CAD build for the part. Positions are in the model's coordinates, mm. A direction names the side the tool comes from. Coordinates: 2 decimals unless noted, no trailing zeros. Write each loop counter-clockwise with the first axis right and the second up, starting at its lowest first coordinate (ties: lowest second). Pieces come first, ordered by that corner, then holes.
```python
from build123d import *

# Parameters (mm, degrees)
BOSS_EXTRUDE1_DEPTH = 10
CUT_EXTRUDE1_DEPTH  = 2
LPATTERN1_COUNT     = 3
LPATTERN1_PITCH     = 2


with BuildPart() as part:
    # Sketch2 → Boss-Extrude1 (new body)
    with BuildSketch(Plane.XY):
        with BuildLine():
            Line((12.25, 1), (12.25, 0.55))
            ThreePointArc((12.25, 0.55), (9.194506694, 0.481441826), (6.145163436, 0.275905297))
            ThreePointArc((6.145163436, 0.275905297), (5.566162178, 0.226280663), (4.986761169, 0.181564549))
            ThreePointArc((4.986761169, 0.181564549), (4.817953434, 0), (4.986761169, -0.181564549))
            ThreePointArc((4.986761169, -0.181564549), (5.566162178, -0.226280663), (6.145163436, -0.275905297))
            ThreePointArc((6.145163436, -0.275905297), (9.194506694, -0.481441826), (12.25, -0.55))
            Line((12.25, -0.55), (12.25, -1))
            ThreePointArc((12.25, -1), (9.174322945, -0.93098895), (6.104836564, -0.724094703))
            ThreePointArc((6.104836564, -0.724094703), (3.055493306, -0.518558174), (0, -0.45))
            ThreePointArc((0, -0.45), (-3.055493306, -0.518558174), (-6.104836564, -0.724094703))
            ThreePointArc((-6.104836564, -0.724094703), (-9.174322945, -0.93098895), (-12.25, -1))
            Line((-12.25, -1), (-12.25, -0.55))
            ThreePointArc((-12.25, -0.55), (-9.194506694, -0.481441826), (-6.145163436, -0.275905297))
            ThreePointArc((-6.145163436, -0.275905297), (-5.566162178, -0.226280663), (-4.986761169, -0.181564549))
            ThreePointArc((-4.986761169, -0.181564549), (-4.817953434, 0), (-4.986761169, 0.181564549))
            ThreePointArc((-4.986761169, 0.181564549), (-5.566162178, 0.226280663), (-6.145163436, 0.275905297))
            ThreePointArc((-6.145163436, 0.275905297), (-9.194506694, 0.481441826), (-12.25, 0.55))
            Line((-12.25, 0.55), (-12.25, 1))
            ThreePointArc((-12.25, 1), (-9.174322945, 0.93098895), (-6.104836564, 0.724094703))
            ThreePointArc((-6.104836564, 0.724094703), (-3.055493306, 0.518558174), (0, 0.45))
            ThreePointArc((0, 0.45), (3.055493306, 0.518558174), (6.104836564, 0.724094703))
            ThreePointArc((6.104836564, 0.724094703), (9.174322945, 0.93098895), (12.25, 1))
        make_face()
    extrude(amount=BOSS_EXTRUDE1_DEPTH)

    # Sketch3 → Cut-Extrude1 (cut, symmetric)
    with BuildSketch(Plane(origin=(0, 0, 0), x_dir=(1, 0, 0), z_dir=(0, 1, 0))):
        Polygon((-2, -3.5), (-1.598076211, -5), (-2, -6.5), (-2.401923789, -5), align=None)
    cut_extrude1 = extrude(amount=CUT_EXTRUDE1_DEPTH, both=True, mode=Mode.SUBTRACT)

    # LPattern1: Cut-Extrude1 ×3
    with Locations(*[(i * LPATTERN1_PITCH, 0, 0) for i in range(1, LPATTERN1_COUNT)]):
        add(cut_extrude1, mode=Mode.SUBTRACT)


solid = part.part
```
Item 1: Flat gauge pins, fed straight in: pin 1 Ø6 at (x, z) = (1, 3.5) entering from -Y; pin 2 Ø1.5 at (x, z) = (1.5, 2) entering from +Y; pin 3 Ø3 at (x, z) = (-7, 1.5) entering from +Y. Where does each tip first touch, or does it go through?
Item 2: Saw through at C-C, the plane z = 7.25. Write the cut outline in (x, y).
Item 3: Wall check: line 1 along Y through (x, z) = (-6, 6); line 2 along Y through (x, z) = (-1.75, 2.5); line 3 along Y through (x, z) = (10, 5). Give the ranges that are in metal, low to high.
Item 4: Saw through at D-D, the plane x = -10. Write the cut outline in (y, z).
Item 5: Saw through at A-A, the plane z = 5.75. State how many separate pieces and enclosed holes the cut face has, and give its area (3 significant figures).
Item 6: Two-plate mould, pull along Z, no slides. Class faces 1 (the flat face through (-0.204, 0.006, 4.26)), 2 (the cylindrical face through (-9.237, -0.483, 4.93)), 3 (the flat face through (0, 0, 0)), 4 (the flat face through (-0.2, 0.01, 5.76)): +Z half, -Z half, draft (parallel to the pull), parting line (faces both ways), or undercut.
Item 7: Saw through at B-B, the plane x = 8.5. Write the cut outline in (y, z), and give its area (3 significant figures).
Item 8: Which spindle directions (+Z, -Z, +X, -X, +Y, -Y) get a long thin tool onto all of the face, cutting with end or side? Do faces 5 (the cylindrical face through (9.217, -0.933, 4.93)), 6 (the cylindrical face through (-9.217, 0.933, 4.93)), 7 (the cylindrical face through (5.574, 0.227, 4.93)). Say none if no direction does.
Working result:
1. pin 1: stops at y = -0.57
1. pin 2: stops at y = 0.49
1. pin 3: stops at y = 0.9
2. outline: (-12.25, -1) arc R68.57 ccw to (-6.1, -0.72) arc R68.12 cw to (6.1, -0.72) arc R68.57 ccw to (12.25, -1) - (12.25, -0.55) arc R68.12 cw to (6.15, -0.28) arc R68.57 ccw to (4.99, -0.18) arc R0.18 cw to (4.99, 0.18) arc R68.57 ccw to (6.15, 0.28) arc R68.12 cw to (12.25, 0.55) - (12.25, 1) arc R68.57 ccw to (6.1, 0.72) arc R68.12 cw to (-6.1, 0.72) arc R68.57 ccw to (-12.25, 1) - (-12.25, 0.55) arc R68.12 cw to (-6.15, 0.28) arc R68.57 ccw to (-4.99, 0.18) arc R0.18 cw to (-4.99, -0.18) arc R68.57 ccw to (-6.15, -0.28) arc R68.12 cw to (-12.25, -0.55) - close
3. line 1: y = -0.71 to -0.26, 0.26 to 0.71
3. line 2: y = -0.47 to 0.47
3. line 3: y = -0.96 to -0.51, 0.51 to 0.96
4. outline: (-0.96, 0) - (-0.51, 0) - (-0.51, 10) - (-0.96, 10) - close; (0.51, 0) - (0.96, 0) - (0.96, 10) - (0.51, 10) - close
5. separate pieces: 4
5. enclosed holes: 0
5. area: 22.1 mm2
6. face 1: undercut
6. face 2: draft
6. face 3: -Z half
6. face 4: undercut
7. outline: (-0.9, 0) - (-0.45, 0) - (-0.45, 10) - (-0.9, 10) - close; (0.45, 0) - (0.9, 0) - (0.9, 10) - (0.45, 10) - close
7. area: 9.01 mm2
8. face 5: +Z, -Z, -Y
8. face 6: +Z, -Z, +Y
8. face 7: +Z, -Z, +X
